Part model, mm, in its own coordinate system. A direction names the side the tool comes from. Coordinates: 2 decimals unless noted, no trailing zeros. Loops run counter-clockwise (first coordinate to the right, second up) from the corner with the lowest first, then second, coordinate; pieces in that order, holes last. Notation, with made-up numbers: (-15.75, -6) -> (36.25, -6) arc R8 ccw to (36.25, 0) -> close; hole circle Ø3 at (26.25, 35.25). An arc over 180 degrees is marked (long way). Use one line per item in the form item = value. Start each with the question number.
(1) Band-saw the part on C-C on z = -15. Count the separate pieces of the cut face and the enclosed holes in it, then the cut area to 3 significant figures.
(2) Band-saw the part on D-D on y = 22. Give the cut face in (x, z).
(3) Drill centre lines: L1, parallel to Y at x = 2.45, z = -15; L2, parallel to X at y = 36.5, z = -22.5; L3, parallel to Z at x = 24.5, y = 14. Where is each one in solid material? Low to high. Write a range as [from, to].
(4) Band-saw the part on B-B on y = 14. Give the cut face in (x, z).
(5) Mould opens along Z. For faces 1 (the cylindrical face through (2.03, 28.74, -13.82)), 2 (the flat face through (4, 17, -12)), 3 (the cylindrical face through (2.03, 0.29, -2.55)) say: +Z half, -Z half, draft (parallel to the pull), parting line (faces both ways), or undercut.
(6) 3-axis set-ups, long thin cutter, end or side, ignore diameter. For faces 4 (the flat face through (15, 17, -26)), 5 (the cylindrical face through (16.6, 14.07, -28.03)), 6 (the flat face through (2, 19, -3)), 7 (the flat face through (15, 19, -30)): which of +Z, -Z, +X, -X, +Y, -Y reach the whole face in a straight line?
(7) Band-saw the part on A-A on x = 15. Give the cut face in (y, z).
(8) Pin check, flat tips, straight feed: P1, Ø3, axis at y = 27.66, z = -15, coming from the +X side; P2, Ø4, axis at x = 15, y = 14, coming from the -Z side; P3, Ø10, axis at y = 18.5, z = -6, coming from the -X side; P4, Ø2, axis at y = 10.5, z = -29.5, coming from the +X side. Stop position of each tip, or through.
```python
from build123d import *

# Parameters (mm, degrees)
SKETCH1_W               = 30
SKETCH1_H               = 30
BOSS_EXTRUDE1_DEPTH     = 62
SHELL1_T                = -4
SKETCH2_R               = 1.6
CUT_EXTRUDE1_DEPTH      = 62
SKETCH3_R               = 25
SKETCH3_R_2             = 2
SKETCH3_W               = 22
SKETCH3_H               = 22
BOSS_EXTRUDE2_DEPTH     = 4
CIRPATTERN1_COUNT       = 2
CIRPATTERN1_ANGLE       = 90
CHAMFER1_SIZE           = 5
FILLET1_R               = 1
FILLET2_R               = 1
SKETCH4_W               = 1.02
SKETCH4_H               = 0.51
CUT_EXTRUDE2_DEPTH      = 83.097503007
CIRPATTERN2_COUNT       = 2
CIRPATTERN2_ANGLE       = 90
SKETCH5_W               = 22
SKETCH5_H               = 14.914082391
CUT_EXTRUDE3_DEPTH      = 87.925255248
CUT_EXTRUDE4_DEPTH      = 84.928541203
CUT_EXTRUDE4_DEPTH_BACK = 84.928541203
SKETCH6_W               = 20
SKETCH6_H               = 15
SKETCH7_W               = 20
SKETCH7_H               = 15
CUT_EXTRUDE5_DEPTH      = 83.743569886
FILLET4_R               = 1
SKETCH8_W               = 39.694573315
SKETCH8_H               = 24
CUT_EXTRUDE6_DEPTH      = 84.928541203
FILLET5_R               = 1


with BuildPart() as part:
    # Sketch1 → Boss-Extrude1 (new body)
    with BuildSketch(Plane(origin=(0, 0, 0), x_dir=(1, 0, 0), z_dir=(0, 1, 0))):
        with Locations((15, 15)):
            Rectangle(SKETCH1_W, SKETCH1_H)
    extrude(amount=BOSS_EXTRUDE1_DEPTH)

    # Shell1
    shell1_openings = [part.faces().sort_by_distance(p)[0] for p in [
        (15, 62, -15),
        (15, 0, -15),
    ]]
    offset(amount=SHELL1_T, openings=shell1_openings, kind=Kind.INTERSECTION)

    # Sketch2 → Cut-Extrude1 (cut)
    with BuildSketch(Plane(origin=(30, 0, 0), x_dir=(0, 0, -1), z_dir=(1, 0, 0))):
        with Locations((15, 14)):
            Circle(SKETCH2_R)
        with Locations((15, 27.66)):
            Circle(SKETCH2_R)
    cut_extrude1 = extrude(amount=-CUT_EXTRUDE1_DEPTH, mode=Mode.SUBTRACT)

    # Sketch3 → Boss-Extrude2 (add)
    with BuildSketch(Plane.XZ):
        with Locations(Location((15, -15, 0), (0, 0, 270))):
            Circle(SKETCH3_R)
        with Locations(Location((34.75, -15, 0), (0, 0, 270))):
            Circle(SKETCH3_R_2, mode=Mode.SUBTRACT)
        with Locations(Location((15, -34.75, 0), (0, 0, 270))):
            Circle(SKETCH3_R_2, mode=Mode.SUBTRACT)
        with Locations(Location((-4.75, -15, 0), (0, 0, 270))):
            Circle(SKETCH3_R_2, mode=Mode.SUBTRACT)
        with Locations(Location((15, 4.75, 0), (0, 0, 270))):
            Circle(SKETCH3_R_2, mode=Mode.SUBTRACT)
        with Locations((15, -15)):
            Rectangle(SKETCH3_W, SKETCH3_H, mode=Mode.SUBTRACT)
    extrude(amount=BOSS_EXTRUDE2_DEPTH)

    # CirPattern1: Cut-Extrude1 ×2 about axis
    cirpattern1_axis = Axis((15, -4, -15), (0, 1, 0))
    for i in range(1, CIRPATTERN1_COUNT):
        add(cut_extrude1.rotate(cirpattern1_axis, i * CIRPATTERN1_ANGLE / (CIRPATTERN1_COUNT - 1)), mode=Mode.SUBTRACT)

    # Chamfer1
    chamfer1_edges = [part.edges().sort_by_distance(p)[0] for p in [
        (0, 31, -30),
        (30, 31, -30),
        (30, 31, 0),
        (0, 31, 0),
    ]]
    chamfer(chamfer1_edges, length=CHAMFER1_SIZE)

    # Fillet1
    # the kernel refuses this fillet: 1 mm, written as the material it takes off along each edge
    with BuildSketch(Plane(origin=(4, 62, -4), x_dir=(-1, 0, 0), z_dir=(0, 0, -1)), Plane(origin=(26, 62, -4), x_dir=(0, 0, 1), z_dir=(-1, 0, 0)), Plane(origin=(26, 62, -26), x_dir=(1, 0, 0), z_dir=(0, 0, 1)), Plane(origin=(4, 62, -26), x_dir=(0, 0, -1), z_dir=(1, 0, 0))) as fillet1_piece_1:
        with BuildLine():
            CenterArc((FILLET1_R, -FILLET1_R), FILLET1_R, 90, 90)
            Line((0, -FILLET1_R), (0, 0))
            Line((0, 0), (FILLET1_R, 0))
        make_face()
    extrude(amount=22, mode=Mode.SUBTRACT)
    with BuildSketch(Plane(origin=(2.5, 62, 0), x_dir=(0, -1, 0), z_dir=(1, 0, 0))) as fillet1_piece_2:
        with BuildLine():
            CenterArc((FILLET1_R, FILLET1_R), FILLET1_R, 180, 90)
            Line((0, FILLET1_R), (0, 0))
            Line((0, 0), (FILLET1_R, 0))
        make_face()
    extrude(amount=25, mode=Mode.SUBTRACT)
    with BuildSketch(Plane(origin=(0, 62, -27.5), x_dir=(1, 0, 0), z_dir=(0, 0, 1)), Plane(origin=(30, 62, -2.5), x_dir=(-1, 0, 0), z_dir=(0, 0, -1)), Plane(origin=(27.5, 62, -30), x_dir=(0, 0, 1), z_dir=(-1, 0, 0))) as fillet1_piece_3:
        with BuildLine():
            CenterArc((FILLET1_R, -FILLET1_R), FILLET1_R, 90, 90)
            Line((0, -FILLET1_R), (0, 0))
            Line((0, 0), (FILLET1_R, 0))
        make_face()
    extrude(amount=25, mode=Mode.SUBTRACT)
    with BuildSketch(Plane(origin=(-1.767766953, 62, -23.232233047), x_dir=(0.7071067811865476, 0, 0.7071067811865476), z_dir=(0.7071067811865476, 0, -0.7071067811865476)), Plane(origin=(23.232233047, 62, 1.767766953), x_dir=(0, -1, 0), z_dir=(0.7071067811865476, 0, -0.7071067811865476))) as fillet1_piece_4:
        with BuildLine():
            CenterArc((FILLET1_R, FILLET1_R), FILLET1_R, 180, 90)
            Line((0, FILLET1_R), (0, 0))
            Line((0, 0), (FILLET1_R, 0))
        make_face()
    extrude(amount=12.071067812, mode=Mode.SUBTRACT)
    with BuildSketch(Plane(origin=(31.767766953, 62, -23.232233047), x_dir=(-0.7071067811865476, 0, 0.7071067811865476), z_dir=(-0.7071067811865476, 0, -0.7071067811865476)), Plane(origin=(6.767766953, 62, 1.767766953), x_dir=(0, -1, 0), z_dir=(-0.7071067811865476, 0, -0.7071067811865476))) as fillet1_piece_5:
        with BuildLine():
            CenterArc((FILLET1_R, -FILLET1_R), FILLET1_R, 90, 90)
            Line((0, -FILLET1_R), (0, 0))
            Line((0, 0), (FILLET1_R, 0))
        make_face()
    extrude(amount=12.071067812, mode=Mode.SUBTRACT)
    with BuildSketch(Plane(origin=(26, 62, -4), x_dir=(0, 0, 1), z_dir=(-1, 0, 0))) as fillet1_piece_6a_section:
        with BuildLine():
            CenterArc((FILLET1_R, -FILLET1_R), FILLET1_R, 90, 90)
            Line((0, -FILLET1_R), (0, 0))
            Line((0, 0), (FILLET1_R, 0))
        make_face()
    fillet1_piece_6a = extrude(amount=24.5, mode=Mode.PRIVATE)
    fillet1_piece_6a = split(fillet1_piece_6a, bisect_by=Plane(origin=(4, 61.773604886, -3.773604886), z_dir=(-1, 0, 0)), keep=Keep.TOP, mode=Mode.PRIVATE)
    with BuildSketch(Plane(origin=(4, 62, -1.5), x_dir=(-1, 0, 0), z_dir=(0, 0, -1))) as fillet1_piece_6b_section:
        with BuildLine():
            CenterArc((FILLET1_R, -FILLET1_R), FILLET1_R, 90, 90)
            Line((0, -FILLET1_R), (0, 0))
            Line((0, 0), (FILLET1_R, 0))
        make_face()
    fillet1_piece_6b = extrude(amount=24.5, mode=Mode.PRIVATE)
    fillet1_piece_6b = split(fillet1_piece_6b, bisect_by=Plane(origin=(3.773604886, 61.773604886, -4), z_dir=(0, 0, 1)), keep=Keep.TOP, mode=Mode.PRIVATE)
    fillet1_piece_6 = fillet1_piece_6a & fillet1_piece_6b
    add(fillet1_piece_6, mode=Mode.SUBTRACT)
    with BuildSketch(Plane(origin=(4, 62, -4), x_dir=(-1, 0, 0), z_dir=(0, 0, -1))) as fillet1_piece_7a_section:
        with BuildLine():
            CenterArc((FILLET1_R, -FILLET1_R), FILLET1_R, 90, 90)
            Line((0, -FILLET1_R), (0, 0))
            Line((0, 0), (FILLET1_R, 0))
        make_face()
    fillet1_piece_7a = extrude(amount=24.5, mode=Mode.PRIVATE)
    fillet1_piece_7a = split(fillet1_piece_7a, bisect_by=Plane(origin=(3.773604886, 61.773604886, -26), z_dir=(0, 0, -1)), keep=Keep.TOP, mode=Mode.PRIVATE)
    with BuildSketch(Plane(origin=(1.5, 62, -26), x_dir=(0, 0, -1), z_dir=(1, 0, 0))) as fillet1_piece_7b_section:
        with BuildLine():
            CenterArc((FILLET1_R, -FILLET1_R), FILLET1_R, 90, 90)
            Line((0, -FILLET1_R), (0, 0))
            Line((0, 0), (FILLET1_R, 0))
        make_face()
    fillet1_piece_7b = extrude(amount=24.5, mode=Mode.PRIVATE)
    fillet1_piece_7b = split(fillet1_piece_7b, bisect_by=Plane(origin=(4, 61.773604886, -26.226395114), z_dir=(-1, 0, 0)), keep=Keep.TOP, mode=Mode.PRIVATE)
    fillet1_piece_7 = fillet1_piece_7a & fillet1_piece_7b
    add(fillet1_piece_7, mode=Mode.SUBTRACT)
    with BuildSketch(Plane(origin=(28.5, 62, -4), x_dir=(0, 0, 1), z_dir=(-1, 0, 0))) as fillet1_piece_8a_section:
        with BuildLine():
            CenterArc((FILLET1_R, -FILLET1_R), FILLET1_R, 90, 90)
            Line((0, -FILLET1_R), (0, 0))
            Line((0, 0), (FILLET1_R, 0))
        make_face()
    fillet1_piece_8a = extrude(amount=24.5, mode=Mode.PRIVATE)
    fillet1_piece_8a = split(fillet1_piece_8a, bisect_by=Plane(origin=(26, 61.773604886, -3.773604886), z_dir=(1, 0, 0)), keep=Keep.TOP, mode=Mode.PRIVATE)
    with BuildSketch(Plane(origin=(26, 62, -26), x_dir=(1, 0, 0), z_dir=(0, 0, 1))) as fillet1_piece_8b_section:
        with BuildLine():
            CenterArc((FILLET1_R, -FILLET1_R), FILLET1_R, 90, 90)
            Line((0, -FILLET1_R), (0, 0))
            Line((0, 0), (FILLET1_R, 0))
        make_face()
    fillet1_piece_8b = extrude(amount=24.5, mode=Mode.PRIVATE)
    fillet1_piece_8b = split(fillet1_piece_8b, bisect_by=Plane(origin=(26.226395114, 61.773604886, -4), z_dir=(0, 0, 1)), keep=Keep.TOP, mode=Mode.PRIVATE)
    fillet1_piece_8 = fillet1_piece_8a & fillet1_piece_8b
    add(fillet1_piece_8, mode=Mode.SUBTRACT)
    with BuildSketch(Plane(origin=(4, 62, -26), x_dir=(0, 0, -1), z_dir=(1, 0, 0))) as fillet1_piece_9a_section:
        with BuildLine():
            CenterArc((FILLET1_R, -FILLET1_R), FILLET1_R, 90, 90)
            Line((0, -FILLET1_R), (0, 0))
            Line((0, 0), (FILLET1_R, 0))
        make_face()
    fillet1_piece_9a = extrude(amount=24.5, mode=Mode.PRIVATE)
    fillet1_piece_9a = split(fillet1_piece_9a, bisect_by=Plane(origin=(26, 61.773604886, -26.226395114), z_dir=(1, 0, 0)), keep=Keep.TOP, mode=Mode.PRIVATE)
    with BuildSketch(Plane(origin=(26, 62, -28.5), x_dir=(1, 0, 0), z_dir=(0, 0, 1))) as fillet1_piece_9b_section:
        with BuildLine():
            CenterArc((FILLET1_R, -FILLET1_R), FILLET1_R, 90, 90)
            Line((0, -FILLET1_R), (0, 0))
            Line((0, 0), (FILLET1_R, 0))
        make_face()
    fillet1_piece_9b = extrude(amount=24.5, mode=Mode.PRIVATE)
    fillet1_piece_9b = split(fillet1_piece_9b, bisect_by=Plane(origin=(26.226395114, 61.773604886, -26), z_dir=(0, 0, -1)), keep=Keep.TOP, mode=Mode.PRIVATE)
    fillet1_piece_9 = fillet1_piece_9a & fillet1_piece_9b
    add(fillet1_piece_9, mode=Mode.SUBTRACT)

    # Fillet2
    fillet2_edges = [part.edges().sort_by_distance(p)[0] for p in [
        (34.75, 0, -13),
        (15, 0, -32.75),
        (-4.75, 0, -13),
        (15, 0, 6.75),
        (15, 0, 10),
        (15, 0, 0),
        (0, 0, -15),
        (30, 0, -15),
        (15, 0, -30),
        (2.5, 0, -2.5),
        (27.5, 0, -2.5),
        (27.5, 0, -27.5),
        (2.5, 0, -27.5),
    ]]
    fillet(fillet2_edges, radius=FILLET2_R)

    # Sketch4 → Cut-Extrude2 (cut, symmetric)
    with BuildSketch(Plane(origin=(4, 0, 0), x_dir=(0, 0, -1), z_dir=(1, 0, 0))):
        with Locations((8.65, 3.205)):
            Rectangle(SKETCH4_W, SKETCH4_H)
        with Locations((21.35, 3.205)):
            Rectangle(SKETCH4_W, SKETCH4_H)
    cut_extrude2 = extrude(amount=CUT_EXTRUDE2_DEPTH, both=True, mode=Mode.SUBTRACT)

    # CirPattern2: Cut-Extrude2 ×2 about axis
    cirpattern2_axis = Axis((15, -4, -15), (0, -1, 0))
    for i in range(1, CIRPATTERN2_COUNT):
        add(cut_extrude2.rotate(cirpattern2_axis, i * CIRPATTERN2_ANGLE / (CIRPATTERN2_COUNT - 1)), mode=Mode.SUBTRACT)

    # Sketch5 → Cut-Extrude3 (cut, through all)
    with BuildSketch(Plane(origin=(0, 62, 0), x_dir=(1, 0, 0), z_dir=(0, 1, 0))):
        with Locations((15, -3.457041196)):
            Rectangle(SKETCH5_W, SKETCH5_H)
    extrude(amount=-CUT_EXTRUDE3_DEPTH, mode=Mode.SUBTRACT)

    # Sketch6 → Cut-Extrude4 (cut, two sides: drawn at the far end of the back side and taken through both)
    with BuildSketch(Plane.ZY.offset(-CUT_EXTRUDE4_DEPTH_BACK)):
        with Locations((-15, 50.5)):
            Rectangle(SKETCH6_W, SKETCH6_H)
    extrude(amount=CUT_EXTRUDE4_DEPTH + CUT_EXTRUDE4_DEPTH_BACK, mode=Mode.SUBTRACT)

    # Sketch7 → Cut-Extrude5 (cut, through all)
    with BuildSketch(Plane(origin=(0, 0, -30), x_dir=(-1, 0, 0), z_dir=(0, 0, -1))):
        with Locations((-15, 50.5)):
            Rectangle(SKETCH7_W, SKETCH7_H)
    extrude(amount=-CUT_EXTRUDE5_DEPTH, mode=Mode.SUBTRACT)

    # Fillet4
    fillet4_edges = [part.edges().sort_by_distance(p)[0] for p in [
        (2, 58, -25),
        (28, 58, -25),
        (2, 43, -5),
        (28, 43, -5),
        (2, 58, -5),
        (2, 43, -25),
        (28, 43, -25),
        (28, 58, -5),
        (25, 43, -28),
        (25, 58, -28),
        (5, 58, -28),
        (5, 43, -28),
    ]]
    fillet(fillet4_edges, radius=FILLET4_R)

    # Sketch8 → Cut-Extrude6 (cut, through all)
    with BuildSketch(Plane.ZY):
        with Locations((-14.809156122, 50)):
            Rectangle(SKETCH8_W, SKETCH8_H)
    extrude(amount=-CUT_EXTRUDE6_DEPTH, mode=Mode.SUBTRACT)

    # Fillet5
    fillet5_edges = [part.edges().sort_by_distance(p)[0] for p in [
        (26, 17, -26),
        (4, 17, -26),
    ]]
    fillet(fillet5_edges, radius=FILLET5_R)


solid = part.part
```
A:
q1.separate_pieces = 8
q1.enclosed_holes = 0
q1.area = 332 mm²
q2.outline = (0, -25) -> (5, -30) -> (25, -30) -> (30, -25) -> (30, -5) -> (26, -1) -> (26, -25) arc R1 cw to (25, -26) -> (5, -26) arc R1 cw to (4, -25) -> (4, -1) -> (0, -5) -> close
q3.L1 = [-4, 12.4], [15.6, 26.06], [29.26, 38]
q3.L2 = [0, 4], [26, 30]
q3.L3 = [-30, -26]
q4.outline = (0, -25) -> (5, -30) -> (13.4, -30) -> (13.4, -26) -> (5, -26) arc R1 cw to (4, -25) -> (4, -16.6) -> (0, -16.6) -> close; (0, -13.4) -> (4, -13.4) -> (4, -1) -> (0, -5) -> close; (16.6, -30) -> (25, -30) -> (30, -25) -> (30, -16.6) -> (26, -16.6) -> (26, -25) arc R1 cw to (25, -26) -> (16.6, -26) -> close; (26, -13.4) -> (30, -13.4) -> (30, -5) -> (26, -1) -> close
q5.face_1 = undercut
q5.face_2 = draft
q5.face_3 = +Z half
q6.face_4 = +Z, +Y, -Y
q6.face_5 = +Z, -Z
q6.face_6 = +Z, -X, +Y
q6.face_7 = -Z, +X, -X, +Y
q7.outline = (-4, -40) -> (-1, -40) arc R1 ccw to (0, -39) -> (0, -37.75) arc R1 ccw to (-1, -36.75) -> (-4, -36.75) -> close; (-4, -32.75) -> (-1, -32.75) arc R1 ccw to (0, -31.75) -> (0, -31) arc R1 cw to (1, -30) -> (12.4, -30) -> (12.4, -26) -> (-4, -26) -> close; (15.6, -30) -> (26.06, -30) -> (26.06, -26) -> (15.6, -26) -> close; (29.26, -30) -> (38, -30) -> (38, -26) -> (29.26, -26) -> close
q8.P1 = through
q8.P2 = -30
q8.P3 = 0
q8.P4 = 26.5
